The model under review builds one solid part; all positions refer to its coordinate system, in mm. A direction names the side the tool comes from. Round coordinates to 2 decimals unless told otherwise and drop trailing zeros. Loops run counter-clockwise (first coordinate to the right, second up) from the corner with the lowest first, then second, coordinate; pieces in that order, holes last. Notation, with made-up numbers: (36.5, -13) -> (56.5, -13) arc R30 cw to (56.5, 18) -> close; hole circle Ø9 at (16, -16.5). An arc over 180 degrees is marked (long way). Use CSV: the item, a comma, the result in double quotes. Start each with the question number.
```python
from build123d import *

# Parameters (mm, degrees)
SKETCH1_W           = 63.22
SKETCH1_H           = 72.35
BOSS_EXTRUDE1_DEPTH = 9.06
CUT_EXTRUDE1_REACH  = 98.506
CUT_EXTRUDE2_REACH  = 98.506
SKETCH3_W           = 6.25
SKETCH3_H           = 17.475
CUT_EXTRUDE3_DEPTH  = 4.185
CUT_EXTRUDE4_START  = -72.35
CUT_EXTRUDE4_DEPTH  = 4.185
CUT_EXTRUDE6_REACH  = 98.506
CUT_EXTRUDE7_REACH  = 94.532
CUT_EXTRUDE8_REACH  = 98.506
SKETCH9_R           = 3.175
SKETCH9_3_R         = 3.175
CUT_EXTRUDE9_DEPTH  = 4.3


with BuildPart() as part:
    # Sketch1 → Boss-Extrude1 (new body)
    with BuildSketch(Plane(origin=(0, 0, 0), x_dir=(1, 0, 0), z_dir=(0, 1, 0))):
        with Locations((-31.61, -36.175)):
            Rectangle(SKETCH1_W, SKETCH1_H)
    extrude(amount=BOSS_EXTRUDE1_DEPTH)

    # Sketch2 → Cut-Extrude1 (cut, up to next)
    with BuildSketch(Plane.XY.offset(72.35), mode=Mode.PRIVATE) as cut_extrude1_sk1:
        Polygon((-63.22, 9.06), (-57.92, 9.06), (-63.22, 0), align=None)
    cut_extrude1_tool1 = extrude(cut_extrude1_sk1.sketch, amount=-CUT_EXTRUDE1_REACH, mode=Mode.PRIVATE) & part.part
    add(cut_extrude1_tool1.solids().sort_by_distance((-61.453333, 6.04, 72.35))[0], mode=Mode.SUBTRACT)

    # Sketch3 → Cut-Extrude2 (cut, up to next)
    with BuildSketch(Plane.XZ, mode=Mode.PRIVATE) as cut_extrude2_sk1:
        with Locations((-60.095, 63.6125)):
            Rectangle(SKETCH3_W, SKETCH3_H)
    cut_extrude2_tool1 = extrude(cut_extrude2_sk1.sketch, amount=-CUT_EXTRUDE2_REACH, mode=Mode.PRIVATE) & part.part
    # Sketch3 → Cut-Extrude2 (cut, up to next)
    with BuildSketch(Plane.XZ, mode=Mode.PRIVATE) as cut_extrude2_sk2:
        with Locations((-60.095, 8.7375)):
            Rectangle(SKETCH3_W, SKETCH3_H)
    cut_extrude2_tool2 = extrude(cut_extrude2_sk2.sketch, amount=-CUT_EXTRUDE2_REACH, mode=Mode.PRIVATE) & part.part
    add(cut_extrude2_tool1.solids().sort_by_distance((-60.095, 0, 63.6125))[0], mode=Mode.SUBTRACT)
    add(cut_extrude2_tool2.solids().sort_by_distance((-60.095, 0, 8.7375))[0], mode=Mode.SUBTRACT)

    # Sketch4 → Cut-Extrude3 (cut)
    with BuildSketch(Plane.XY.offset(72.35)):
        Polygon((-56.97, 9.06), (-56.97, 4.06), (-26.97, 7.21), (-26.97, 9.06), align=None)
    extrude(amount=-CUT_EXTRUDE3_DEPTH, mode=Mode.SUBTRACT)

    # Sketch4<2> → Cut-Extrude4 (cut)
    with BuildSketch(Plane.XY.offset(72.35).offset(CUT_EXTRUDE4_START)):
        Polygon((-56.97, 9.06), (-56.97, 4.06), (-26.97, 7.21), (-26.97, 9.06), align=None)
    extrude(amount=CUT_EXTRUDE4_DEPTH, mode=Mode.SUBTRACT)

    # Sketch7 → Cut-Extrude6 (cut, up to next)
    with BuildSketch(Plane.XY.offset(72.35), mode=Mode.PRIVATE) as cut_extrude6_sk1:
        Polygon((0, 0), (-4, 9.06), (0, 9.06), align=None)
    cut_extrude6_tool1 = extrude(cut_extrude6_sk1.sketch, amount=-CUT_EXTRUDE6_REACH, mode=Mode.PRIVATE) & part.part
    add(cut_extrude6_tool1.solids().sort_by_distance((-1.333333, 6.04, 72.35))[0], mode=Mode.SUBTRACT)

    # Sketch8 → Cut-Extrude7 (cut, up to next)
    with BuildSketch(Plane.ZY.offset(56.97), mode=Mode.PRIVATE) as cut_extrude7_sk1:
        Polygon((72.35, 0), (71.01, 0), (72.35, 9.06), align=None)
    cut_extrude7_tool1 = extrude(cut_extrude7_sk1.sketch, amount=-CUT_EXTRUDE7_REACH, mode=Mode.PRIVATE) & part.part
    # Sketch8 → Cut-Extrude7 (cut, up to next)
    with BuildSketch(Plane.ZY.offset(56.97), mode=Mode.PRIVATE) as cut_extrude7_sk2:
        Polygon((0, 0), (1.34, 0), (0, 9.06), align=None)
    cut_extrude7_tool2 = extrude(cut_extrude7_sk2.sketch, amount=-CUT_EXTRUDE7_REACH, mode=Mode.PRIVATE) & part.part
    add(cut_extrude7_tool1.solids().sort_by_distance((-56.97, 3.02, 71.903333))[0], mode=Mode.SUBTRACT)
    add(cut_extrude7_tool2.solids().sort_by_distance((-56.97, 3.02, 0.446667))[0], mode=Mode.SUBTRACT)

    # Sketch9 → Cut-Extrude8 (cut, up to next)
    with BuildSketch(Plane.XZ, mode=Mode.PRIVATE) as cut_extrude8_sk1:
        with Locations(Location((-25.415, 36.175, 0), (0, 0, 270))):
            Circle(SKETCH9_R)
    cut_extrude8_tool1 = extrude(cut_extrude8_sk1.sketch, amount=-CUT_EXTRUDE8_REACH, mode=Mode.PRIVATE) & part.part
    add(cut_extrude8_tool1.solids().sort_by_distance((-25.415, 0, 36.175))[0], mode=Mode.SUBTRACT)

    # Sketch9<3> → Cut-Extrude9 (cut)
    with BuildSketch(Plane.XZ):
        Polygon((-22.269171962, 41.691982807), (-28.619933244, 41.6578584), (-31.765761282, 36.140875593), (-28.560828038, 30.658017193), (-22.210066756, 30.6921416), (-19.064238718, 36.209124407), align=None)
        with Locations(Location((-25.415, 36.175, 0), (0, 0, 270))):
            Circle(SKETCH9_3_R, mode=Mode.SUBTRACT)
    extrude(amount=-CUT_EXTRUDE9_DEPTH, mode=Mode.SUBTRACT)


solid = part.part
```
1. Take a section at D-D, the plane z = 21.5. Give the boundary of the cut face in (x, y).
2. For line 1 along Y through (x, z) = (-29, 32); line 2 along Y through (x, z) = (-59, 46.5); line 3 along Z through (x, y) = (-58, 3.25) (3 decimals), list the stretches that pass through material, from the lowest coordinate up. Write a range as from..to.
3. Take a section at C-C, the plane x = -36.5. Give the boundary of the cut face in (y, z) (3 decimals).
4. Clearance check with flat-ended pins moving along their axes: P1, Ø1.5, axis at y = 3.5, z = 23.5, coming from the -X side; P2, Ø3, axis at y = 1, z = 21, coming from the +X side; P3, Ø2.5, axis at y = 7, z = 8.5, coming from the -X side; P4, Ø5, axis at x = -25.415, z = 36.175, coming from the -Y side. State where each tip first meets the part, or that it passes through.
5. Take a section at B-B, the plane y = 5.75. Give the boundary of the cut face in (x, z) (3 decimals), then the cut area to 3 significant figures.
6. For faces 4 (the face through (-30.186, 2.12, 33.438)), 5 (the face through (-42.18, 5.613, 2.202)), 6 (the face through (-26.97, 8, 70)), list the 3-axis set-ups (+Z, -Z, +X, -X, +Y, -Y) from which the entire face can be reached by the end or side of a thin tool; tool diameter is ignored.
7. The part is to be moulded in two halves that separate along Z. For faces 1 (the face through (-23, 4.3, 39)), 2 (the face through (-59, 3, 17.475)), 3 (the face through (-60.533, 4.593, 36.437)), say which applies: pulls with the +Z half, pulls with the -Z half, needs draft (parallel to the pull), parting line crosses it, or undercut.
8. Take a section at A-A, the plane z = 38. Give the boundary of the cut face in (x, y), then the cut area to 3 significant figures.
Results:
1,outline,"(-63.22, 0) -> (0, 0) -> (-4, 9.06) -> (-57.92, 9.06) -> close"
2,line 1,"4.3..9.06"
2,line 2,"0..7.21"
2,line 3,"17.475..54.875"
3,outline,"(0, 1.34) -> (6.209, 0.422) -> (6.209, 4.185) -> (9.06, 4.185) -> (9.06, 68.165) -> (6.209, 68.165) -> (6.209, 71.928) -> (0, 71.01) -> close"
4,P1,"x = -61.61"
4,P2,"x = 0"
4,P3,"x = -56.97"
4,P4,"through"
5,outline,"(-59.856, 17.475) -> (-56.97, 17.475) -> (-56.97, 4.185) -> (-40.875, 4.185) -> (-40.875, 0.49) -> (-2.539, 0.49) -> (-2.539, 71.86) -> (-40.875, 71.86) -> (-40.875, 68.165) -> (-56.97, 68.165) -> (-56.97, 54.875) -> (-59.856, 54.875) -> close; hole circle Ø6.35 at (-25.415, 36.175)"
5,area,"3,840 mm²"
6,face 4,"-Y"
6,face 5,"-Z, -X, +Y"
6,face 6,"+Z, -X, +Y"
7,face 1,"undercut"
7,face 2,"pulls with the -Z half"
7,face 3,"needs draft"
8,outline,"(-63.22, 0) -> (-30.71, 0) -> (-30.71, 4.3) -> (-28.01, 4.3) -> (-28.01, 9.06) -> (-57.92, 9.06) -> close; (-22.82, 4.3) -> (-20.11, 4.3) -> (-20.11, 0) -> (0, 0) -> (-4, 9.06) -> (-22.82, 9.06) -> close"
8,area,"460 mm²"
